from build123d import *

# Parameters (mm, degrees)
F1_DEPTH = 12
F2_DEPTH = 10


with BuildPart() as f1:
    # F0 (on Top) → F1 (new body)
    with BuildSketch(Plane.XY):
        Polygon((20, 20), (0, 0), (2390, 0), (2370, 20), align=None)
    extrude(amount=F1_DEPTH)

    # F0 (on Top) → F2 (join)
    with BuildSketch(Plane.XY):
        Polygon((30, 30), (20, 20), (2370, 20), (2360, 30), align=None)
    extrude(amount=F2_DEPTH)


with BuildPart() as f3_1:
    # F3: copy of F1
    add(f1.part)


solid = f1.part
Can you work these out from the model? Positions are in its coordinate system, mm. Round coordinates to 2 decimals unless told otherwise and drop trailing zeros. Write each loop counter-clockwise with the first axis right and the second up, starting at its lowest first coordinate (ties: lowest second). Pieces come first, ordered by that corner, then holes. Notation, with made-up numbers: (72, 19.25) - (93, 19.25) arc R31 ccw to (93, 57.25) - close; hole circle Ø10 at (3.5, -30). An arc over 180 degrees is marked (long way). Write each question's results on one line, items separated by ' | '. Start each with the question number.
1) For pin 1 Ø6 at (y, z) = (8.5, 10.5) entering from -X; pin 2 Ø5 at (x, y) = (1273, 24.5) entering from +Z; pin 3 Ø1 at (x, z) = (751.5, 11) entering from +Y, each with a flat end and sliding along its axis, tell me the tip position at first contact or that it passes through.
2) Please list where these lines run through material, in increasing order: line 1 (Z direction, x = 855.5, y = 23.5); line 2 (Y direction, x = 2025.5, z = 10.75); line 3 (X direction, y = 1.5, z = 6.5).
3) Suppose I cut it at A-A (x = 1559). List the corners of the cut face in (y, z) for me.
Here are the results:
1) pin 1: stops at x = 5.5 | pin 2: stops at z = 10 | pin 3: stops at y = 20
2) line 1: z = 0 to 10 | line 2: y = 0 to 20 | line 3: x = 1.5 to 2388.5
3) outline: (0, 0) - (30, 0) - (30, 10) - (20, 10) - (20, 12) - (0, 12) - close
